Job drawing, mm, ordinate dimensions from the low corner. One solid piece. Round coordinates to 2 decimals unless told otherwise and drop trailing zeros. Loops run counter-clockwise (first coordinate to the right, second up) from the corner with the lowest first, then second, coordinate; pieces in that order, holes last. Notation, with made-up numbers: M 85.25,84 L 142.25,84 A17 ccw 142.25,113 Z; hole C 58.25,21.25 d8. An arc over 180 degrees is marked long. Put each result on its own line as item: value. Start each with the question number.
1) Probe line 1 along Y through (x, z) = (116.5, 183). List the from-to ranges inside material, lowest first.
2) Drop flat-ended pins along their axis: pin 1 Ø6.5 at (y, z) = (110.5, 128.5) entering from +X; pin 2 Ø14 at (y, z) = (4.5, 138) entering from -X; pin 3 Ø10 at (x, z) = (27, 39.5) entering from +Y. Give the stop position or say it passes through.
3) Pull direction Y, two halves, no side cores. Call the marked faces 1, 2 and 3: +Y half, -Y half, draft (parallel to the pull), parting line (faces both ways), or undercut.
4) Slice it at B-B on y = 76.5. Give the cut face in (x, z).
5) Slice it at C-C on z = 149.5. Give the cut face in (x, y), then the cut area to 3 significant figures.
6) Slice it at A-A on x = 141. Give the cut face in (y, z).
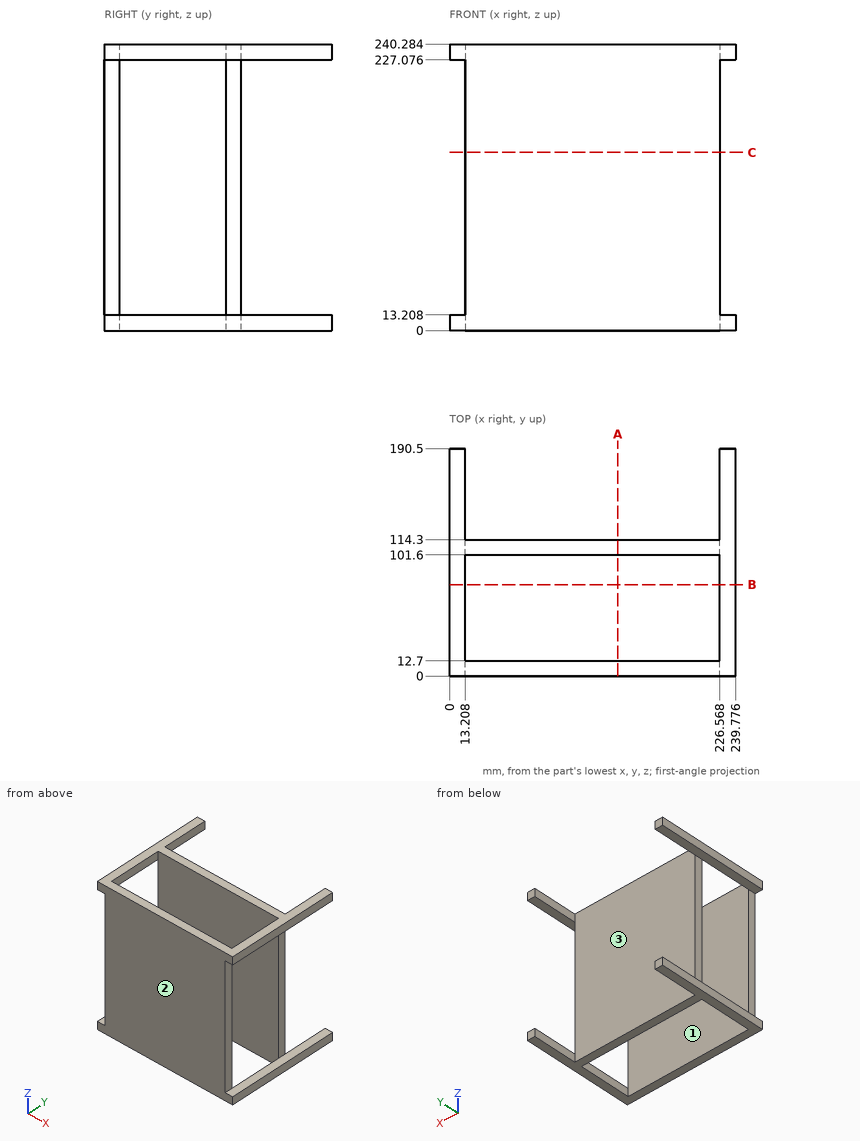
Recorded:
1. line 1: y = 0 to 12.7, 101.6 to 114.3
2. pin 1: stops at x = 226.57
2. pin 2: stops at x = 13.21
2. pin 3: stops at y = 114.3
3. face 1: undercut
3. face 2: -Y half
3. face 3: +Y half
4. outline: M 0,0 L 13.21,0 L 13.21,13.21 L 0,13.21 Z; M 0,227.08 L 13.21,227.08 L 13.21,240.28 L 0,240.28 Z; M 226.57,0 L 239.78,0 L 239.78,13.21 L 226.57,13.21 Z; M 226.57,227.08 L 239.78,227.08 L 239.78,240.28 L 226.57,240.28 Z
5. outline: M 13.21,0 L 226.57,0 L 226.57,12.7 L 13.21,12.7 Z; M 13.21,101.6 L 226.57,101.6 L 226.57,114.3 L 13.21,114.3 Z
5. area: 5,420 mm2
6. outline: M 0,0 L 12.7,0 L 12.7,240.28 L 0,240.28 Z; M 101.6,0 L 114.3,0 L 114.3,240.28 L 101.6,240.28 Z
